Source: CAD feature listing. Evaluate the final solid. Frame: model axes, mm. A direction names the side the tool comes from. Round coordinates to 2 decimals unless told otherwise and drop trailing zeros. Order: outer loops, then holes, each group sorted by start corner. A loop starts at its lowest first (then second) coordinate and runs counter-clockwise, first axis right, second up. Notation, with made-up numbers: M 80.5,2.25 L 117.5,2.25 A29 ccw 117.5,31.25 Z; hole C 76,65.5 d9. An arc over 180 degrees is marked long. Use one line per item in the form item = value. Start each with the question number.
Q1. Pull-direction query (Z, two-part tool) for faces 1 (the cylindrical face through (-9.1, -30.07, 3.14)), 2 (the cylindrical face through (-1.2, -32.9, 5.9)); classes: pulls with the +Z half, pulls with the -Z half, needs draft (parallel to the pull), parting line crosses it, or undercut.
Q2. Reachability of faces 3 (the flat face through (25, -9, 6)), 4 (the flat face through (-10, -25, 6)), 5 (the flat face through (-25, 25, 6)) from +Z, -Z, +X, -X, +Y, -Y: full face, straight path, thin tool, end or side. Return the list, or none.
Q3. Material intervals for probe 1 along Y at (x, z) = (0, 8.25); probe 2 along X at (y, z) = (-29.5, 6.25); probe 3 along X at (y, z) = (-15.5, 10.5), sorted ascending.
Q4. Section A-A (x = 0). Return the cut outline in (y, z), plus the area to 3 significant figures.
Q5. Section C-C (x = -12). Return the cut outline in (y, z), plus the area to 3 significant figures.
Q6. Section D-D (y = -19). Return the cut outline in (x, z), plus the area to 3 significant figures.
Q7. Contact query for flat-ended pins moving along their axis: pin 1 (3 mm diameter, centred on x = -25.5, z = 7.5, fed in from +Y); pin 2 (1.8 mm diameter, centred on y = -27.5, z = 5, fed in from +X); pin 3 (5 mm diameter, centred on x = -8, z = 6, fed in from +Y); pin 4 (1.8 mm diameter, centred on y = -29, z = 7.5, fed in from -X). Output: stop coordinate, or through.
from build123d import *

# Parameters (mm, degrees)
SKETCH_1_W          = 70
SKETCH_1_H          = 70
SKETCH_1_R          = 1.5
SKETCH_1_R_2        = 21
EXTRUDE_1_DEPTH     = 12
SKETCH_3_R          = 3
CUT_EXTRUDE_2_DEPTH = 10
SKETCH_4_R          = 3
CUT_EXTRUDE_3_DEPTH = 10
CUT_EXTRUDE_START   = -10
SKETCH_5_R          = 3
CUT_EXTRUDE_4_DEPTH = 10
SKETCH_6_R          = 3
CUT_EXTRUDE_5_DEPTH = 10


with BuildPart() as part:
    # 草图1 → 凸台-拉伸1 (new body)
    with BuildSketch(Plane.XY):
        Rectangle(SKETCH_1_W, SKETCH_1_H)
        with Locations((32, 0)):
            Circle(SKETCH_1_R, mode=Mode.SUBTRACT)
        with Locations((27.712812921, -16)):
            Circle(SKETCH_1_R, mode=Mode.SUBTRACT)
        with Locations((16, -27.712812921)):
            Circle(SKETCH_1_R, mode=Mode.SUBTRACT)
        with Locations((0, -32)):
            Circle(SKETCH_1_R, mode=Mode.SUBTRACT)
        with Locations((-16, -27.712812921)):
            Circle(SKETCH_1_R, mode=Mode.SUBTRACT)
        with Locations((-27.712812921, -16)):
            Circle(SKETCH_1_R, mode=Mode.SUBTRACT)
        with Locations((-32, 0)):
            Circle(SKETCH_1_R, mode=Mode.SUBTRACT)
        with Locations((-27.712812921, 16)):
            Circle(SKETCH_1_R, mode=Mode.SUBTRACT)
        with Locations((-16, 27.712812921)):
            Circle(SKETCH_1_R, mode=Mode.SUBTRACT)
        with Locations((0, 32)):
            Circle(SKETCH_1_R, mode=Mode.SUBTRACT)
        with Locations((16, 27.712812921)):
            Circle(SKETCH_1_R, mode=Mode.SUBTRACT)
        with Locations((27.712812921, 16)):
            Circle(SKETCH_1_R, mode=Mode.SUBTRACT)
        Circle(SKETCH_1_R_2, mode=Mode.SUBTRACT)
    extrude(amount=EXTRUDE_1_DEPTH)

    # 草图3 → 切除-拉伸2 (cut)
    with BuildSketch(Plane(origin=(0, 35, 0), x_dir=(1, 0, 0), z_dir=(0, 1, 0))):
        with Locations(Location((-25, -6, 0), (0, 0, 270))):
            Circle(SKETCH_3_R)
        with Locations(Location((-8, -6, 0), (0, 0, 270))):
            Circle(SKETCH_3_R)
        with Locations(Location((25, -6, 0), (0, 0, 90))):
            Circle(SKETCH_3_R)
        with Locations(Location((8, -6, 0), (0, 0, 90))):
            Circle(SKETCH_3_R)
    extrude(amount=-CUT_EXTRUDE_2_DEPTH, mode=Mode.SUBTRACT)

    # 草图4 → 切除-拉伸3 (cut)
    with BuildSketch(Plane(origin=(35, 0, 0), x_dir=(0, 0, -1), z_dir=(1, 0, 0))):
        with Locations((-6, -9)):
            Circle(SKETCH_4_R)
        with Locations((-6, -29)):
            Circle(SKETCH_4_R)
    extrude(amount=-CUT_EXTRUDE_3_DEPTH, mode=Mode.SUBTRACT)

    # 草图5 → 切除-拉伸4 (cut)
    with BuildSketch(Plane.ZY.offset(35).offset(CUT_EXTRUDE_START)):
        with Locations(Location((6, -29, 0), (0, 0, 180))):
            Circle(SKETCH_5_R)
        with Locations(Location((6, -9, 0), (0, 0, 180))):
            Circle(SKETCH_5_R)
    extrude(amount=CUT_EXTRUDE_4_DEPTH, mode=Mode.SUBTRACT)

    # 草图6 → 切除-拉伸5 (cut)
    with BuildSketch(Plane.XZ.offset(35)):
        with Locations(Location((10, 6, 0), (0, 0, 270))):
            Circle(SKETCH_6_R)
        with Locations(Location((-10, 6, 0), (0, 0, 270))):
            Circle(SKETCH_6_R)
    extrude(amount=-CUT_EXTRUDE_5_DEPTH, mode=Mode.SUBTRACT)


solid = part.part
Results list:
q1.face_1 = undercut
q1.face_2 = needs draft
q2.face_3 = +X
q2.face_4 = -Y
q2.face_5 = +Y
q3.probe_1 = -35 to -33.5, -30.5 to -21, 21 to 30.5, 33.5 to 35
q3.probe_2 = -25 to -12.99, -7.01 to 7.01, 12.99 to 25
q3.probe_3 = -35 to -29.13, -26.3 to -14.17, 14.17 to 26.3, 29.13 to 35
q4.outline = M -35,0 L -33.5,0 L -33.5,12 L -35,12 Z; M -30.5,0 L -21,0 L -21,12 L -30.5,12 Z; M 21,0 L 30.5,0 L 30.5,12 L 21,12 Z; M 33.5,0 L 35,0 L 35,12 L 33.5,12 Z
q4.area = 264 mm2
q5.outline = M -35,0 L -17.23,0 L -17.23,12 L -35,12 L -35,8.24 L -25,8.24 L -25,3.76 L -35,3.76 Z; M 17.23,0 L 35,0 L 35,12 L 17.23,12 Z
q5.area = 382 mm2
q6.outline = M -35,0 L -8.94,0 L -8.94,12 L -35,12 Z; M 8.94,0 L 35,0 L 35,12 L 8.94,12 Z
q6.area = 625 mm2
q7.pin_1 = 35
q7.pin_2 = 25
q7.pin_3 = 25
q7.pin_4 = -25
